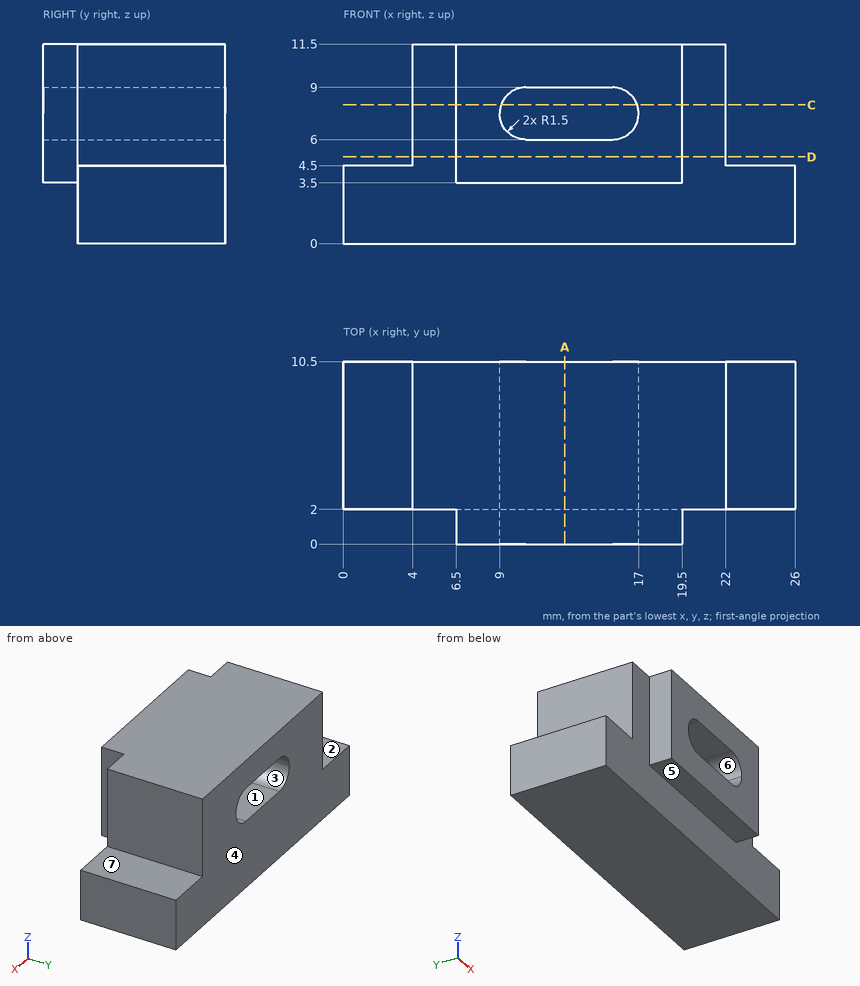
Check sheet for the drawn part. Datum: minimum x, y, z corner. Units: mm. A direction names the side the tool comes from. Coordinates: 2 decimals unless noted, no trailing zeros. Order: outer loops, then holes, each group sorted by start corner. A loop starts at its lowest first (then second) coordinate and runs counter-clockwise, first axis right, second up. Notation, with made-up numbers: M 16,54.5 L 23,54.5 A30 cw 23,79.5 Z; hole C 34,-9 d7. An arc over 180 degrees is marked long. One line per question, with ' | ' between items. Start each with the question number.
Item 1: Gauge pin test, flat ends, axial feed: pin 1 (3 mm diameter, centred on x = 2, y = 5.5, fed in from +Z); pin 2 (1 mm diameter, centred on y = 1, z = 6, fed in from -X); pin 3 (0.6 mm diameter, centred on y = 1, z = 6, fed in from +X). Record the tip position at first contact, or that the pin passes through.
Item 2: Cross-section at C-C on z = 8. Enter the section's corners in (x, y).
Item 3: Cross-section at D-D on z = 5. Enter the section's corners in (x, y), then the cut area to 3 significant figures.
Item 4: Set-up check for the marked faces 5, 6 and 7: record each of +Z, -Z, +X, -X, +Y, -Y from which the full face is reachable in a straight line by a thin tool's end or side.
Item 5: Cross-section at A-A on x = 12.75. Enter the section's corners in (y, z), then the cut area to 4 significant figures.
Item 6: Material ranges on L1, parallel to Z at x = 10.5, y = 9; L2, parallel to Y at x = 14, z = 1.25; L3, parallel to X at y = 5, z = 5.5, recorded low to high. Write a range as [from, to].
Item 7: Draft check along Z on the marked faces 1, 2, 3 and 4. Enter one of: pulls with the +Z half, pulls with the -Z half, needs draft (parallel to the pull), parting line crosses it, or undercut.
Findings:
1) pin 1: stops at z = 4.5 | pin 2: stops at x = 6.5 | pin 3: stops at x = 19.5
2) outline: M 4,2 L 6.5,2 L 6.5,0 L 9.09,0 L 9.09,10.5 L 4,10.5 Z; M 16.91,0 L 19.5,0 L 19.5,2 L 22,2 L 22,10.5 L 16.91,10.5 Z
3) outline: M 4,2 L 6.5,2 L 6.5,0 L 19.5,0 L 19.5,2 L 22,2 L 22,10.5 L 4,10.5 Z | area: 179 mm²
4) face 5: -Z, +X, -X, -Y | face 6: +Y, -Y | face 7: +Z, +X, +Y, -Y
5) outline: M 0,3.5 L 2,3.5 L 2,0 L 10.5,0 L 10.5,6 L 0,6 Z; M 0,9 L 10.5,9 L 10.5,11.5 L 0,11.5 Z | area: 82.25 mm²
6) L1: z = [0, 6], [9, 11.5] | L2: y = [2, 10.5] | L3: x = [4, 22]
7) face 1: undercut | face 2: pulls with the +Z half | face 3: undercut | face 4: needs draft
